The figure shows three views and two pictorial views of one solid part (mm, origin at its lowest corner). Answer the questions. A direction names the side the tool comes from. Round coordinates to 2 decimals unless told otherwise and drop trailing zeros. Loops run counter-clockwise (first coordinate to the right, second up) from the corner with the lowest first, then second, coordinate; pieces in that order, holes last. Notation, with made-up numbers: (-5, 54) -> (29, 54) arc R28 cw to (29, 84) -> close; hole circle Ø11 at (-12, 10.25). An arc over 180 degrees is marked (long way). Put each result on its own line as item: value.
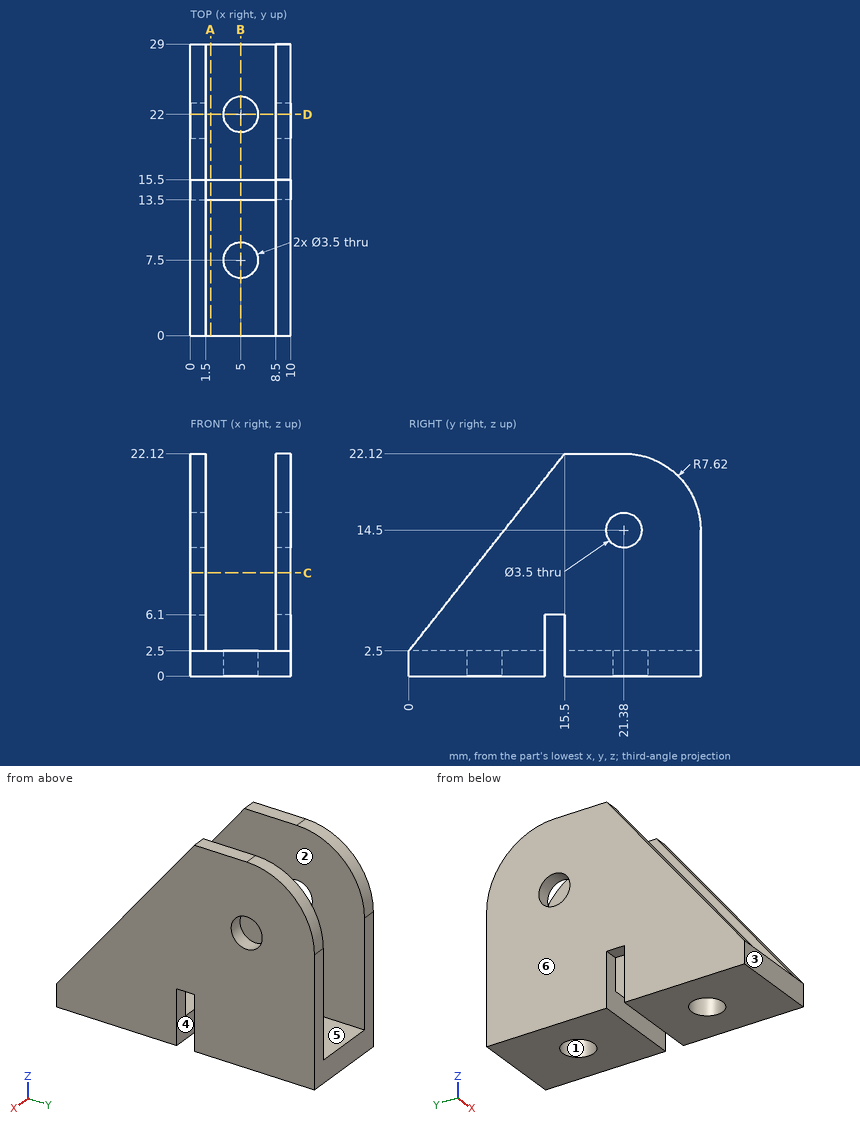
Item 1: The part is cut by section D-D (y = 22). State how many separate pieces and enclosed holes the cut face has, then the cut area to 3 significant figures.
Derived:
separate pieces: 4
enclosed holes: 0
area: 65.2 mm^2
Item 2: The part is cut by section A-A (x = 2). Determine the outline of the cut face in (y, z), then the cut area to 3 significant figures.
Derived:
outline: (0, 0) -> (13.5, 0) -> (13.5, 2.5) -> (0, 2.5) -> close; (15.5, 0) -> (29, 0) -> (29, 2.5) -> (15.5, 2.5) -> close
area: 67.5 mm^2
Item 3: Which of the six approach directions +Z, -Z, +X, -X, +Y, -Y give full straight-line access (tool end or side, diameter ignored) to the marked faces 4, 5 and 6?
Derived:
face 4: -Z, +X, -X
face 5: +Z, +Y, -Y
face 6: +Z, -Z, -X, +Y, -Y
Item 4: The part is cut by section C-C (z = 10.25). Determine the outline of the cut face in (x, y).
Derived:
outline: (0, 6.12) -> (1.5, 6.12) -> (1.5, 29) -> (0, 29) -> close; (8.5, 6.12) -> (10, 6.12) -> (10, 29) -> (8.5, 29) -> close
Item 5: Find the intervals of material crossed by line 1 along Y through (x, z) = (5, 1.85); line 2 along Y through (x, z) = (8, 1.75); line 3 along X through (y, z) = (21.75, 6), in increasing order.
Derived:
line 1: y = 0 to 5.75, 9.25 to 13.5, 15.5 to 20.25, 23.75 to 29
line 2: y = 0 to 13.5, 15.5 to 29
line 3: x = 0 to 1.5, 8.5 to 10
Item 6: The part is cut by section B-B (x = 5). Determine the outline of the cut face in (y, z), then the cut area to 3 significant figures.
Derived:
outline: (0, 0) -> (5.75, 0) -> (5.75, 2.5) -> (0, 2.5) -> close; (9.25, 0) -> (13.5, 0) -> (13.5, 2.5) -> (9.25, 2.5) -> close; (15.5, 0) -> (20.25, 0) -> (20.25, 2.5) -> (15.5, 2.5) -> close; (23.75, 0) -> (29, 0) -> (29, 2.5) -> (23.75, 2.5) -> close
area: 50.0 mm^2
Item 7: Flat-ended cylindrical pins translate along their axes: pin 1 Ø6 at (x, z) = (1.5, 9) entering from -Y (1 decimal); pin 2 Ø1.5 at (x, y) = (3.5, 18) entering from +Z; pin 3 Ø0.5 at (x, y) = (1, 15) entering from -Z. Find the tip coordinate at first contact, or state that the pin passes through.
Derived:
pin 1: stops at y = 2.8
pin 2: stops at z = 2.5
pin 3: stops at z = 6.1
Item 8: For a pull along Y with two mould halves and no side action, classify the marked faces 1, 2 and 3 as pulls with the +Y half, pulls with the -Y half, needs draft (parallel to the pull), parting line crosses it, or undercut.
Derived:
face 1: undercut
face 2: needs draft
face 3: pulls with the -Y half
